Input: part model. Units: mm. Frame: model coordinates. Face numbers are marked on the shaded views. Coordinates: 2 decimals unless noted, no trailing zeros. Loops run counter-clockwise (first coordinate to the right, second up) from the corner with the lowest first, then second, coordinate; pieces in that order, holes last.
Item 1: Section B-B on x = 130.5. Return loops of the section in (y, z) (3 decimals).
Item 2: Section A-A on z = -22. Return loops of the section in (x, y) (3 decimals), and give its area (3 significant figures).
Item 3: Ray query, line 1 along X through (y, z) = (13.75, -50) (3 decimals); line 2 along X through (y, z) = (1.05, 0) (3 decimals); line 3 along Z through (x, y) = (141.5, 22.5) (3 decimals). Return the intervals inside material, ascending.
Item 4: Pull-direction query (X, two-part tool) for the marked faces 1 and 2; classes: released by +X, released by -X, zero draft, split by the parting line, or undercut.
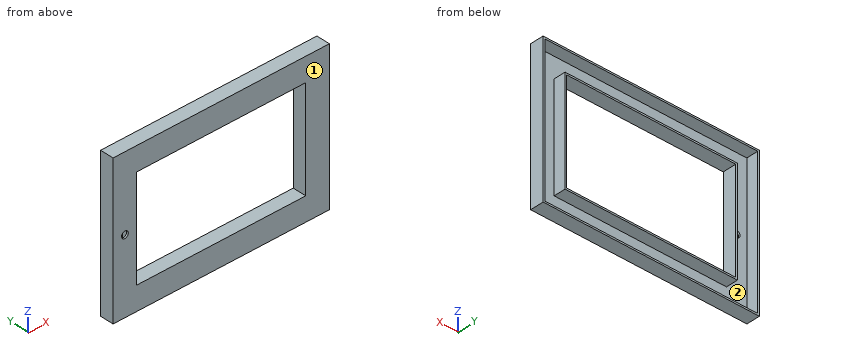
Autodesk Inventor part; units mm, degrees
ref_plane "YZ Plane" through (0, 0, 0) normal (1, 0, 0) x (0, 1, 0)
ref_plane "XZ Plane" through (0, 0, 0) normal (0, 1, 0) x (-1, 0, 0)
ref_plane "XY Plane" through (0, 0, 0) normal (0, 0, 1) x (1, 0, 0)
sketch "Sketch3" plane through (0, 0, 0) normal (0, 1, 0) x (-1, 0, 0)
  line L0 (-203.2, 139.7) -> (203.2, 139.7)
  line L1 (203.2, 139.7) -> (203.2, -139.7)
  line L2 (203.2, -139.7) -> (-203.2, -139.7)
  line L3 (-203.2, -139.7) -> (-203.2, 139.7)
  line L4 (-203.2, 139.7) -> (203.2, -139.7) construction
  line L5 (203.2, 139.7) -> (-203.2, -139.7) construction
  line L6 (152.4, -88.9) -> (152.4, 88.9)
  line L7 (152.4, 88.9) -> (-152.4, 88.9)
  line L8 (-152.4, 88.9) -> (-152.4, -88.9)
  line L9 (-152.4, -88.9) -> (152.4, -88.9)
  line L10 (158.75, -95.25) -> (158.75, 95.25)
  line L11 (158.75, 95.25) -> (-158.75, 95.25)
  line L12 (-158.75, 95.25) -> (-158.75, -95.25)
  line L13 (-158.75, -95.25) -> (158.75, -95.25)
  point P0 (0, 0)
  dimension "d11" = 406.4
  dimension "d12" = 279.4
  dimension "d13" = 50.8
  dimension "d14" = 44.45
extrude "Extrusion3" add sketch "Sketch3" along normal blind 50.8 contours L0 L1 L2 L3
shell "Shell2" thickness 3.175 removed faces 1 at (52.9167, 50.8, -124.8833)
sketch "Sketch4" plane through (0, 50.8, 0) normal (0, 1, 0) x (1, 0, 0)
  line L0 (227.9599, -165.6341) -> (-227.9599, -165.6341)
  line L1 (-227.9599, -165.6341) -> (-227.9599, 165.6341)
  line L2 (-227.9599, 165.6341) -> (227.9599, 165.6341)
  line L3 (227.9599, 165.6341) -> (227.9599, -165.6341)
  line L4 (227.9599, -165.6341) -> (-227.9599, 165.6341) construction
  line L5 (-227.9599, -165.6341) -> (227.9599, 165.6341) construction
  point P0 (0, 0)
extrude "Extrusion4" cut sketch "Sketch4" against normal blind 25.4
sketch "Sketch5" plane through (-200.025, 3.175, 136.525) normal (0, 1, 0) x (1, 0, 0)
  line L0 (361.95, 234.95) -> (38.1, 234.95)
  line L1 (361.95, 38.1) -> (361.95, 234.95)
  line L2 (38.1, 38.1) -> (361.95, 38.1)
  line L3 (38.1, 234.95) -> (38.1, 38.1)
  line L4 (400.05, 0) -> (0, 0)
  line L5 (400.05, 273.05) -> (400.05, 0)
  line L6 (0, 273.05) -> (400.05, 273.05)
  line L7 (0, 0) -> (0, 273.05)
  line L8 (38.1, 38.1) -> (0, 38.1)
  line L9 (0, 38.1) -> (0, 234.95)
  line L10 (0, 234.95) -> (38.1, 234.95)
  line L11 (38.1, 234.95) -> (38.1, 38.1)
  circle A0 centre (19.05, 136.525) radius 6.35
  point P0 (200.025, 136.525)
  dimension "d20" = 12.7
extrude "Extrusion5" cut sketch "Sketch5" against normal blind 25.4 contours A0
properties part number "Catch pan" material "Aluminum 6061"
Results found:
1. outline: (0, -139.7) - (25.4, -139.7) - (25.4, -136.525) - (3.175, -136.525) - (3.175, -98.425) - (25.4, -98.425) - (25.4, -95.25) - (0, -95.25) - close; (0, 95.25) - (25.4, 95.25) - (25.4, 98.425) - (3.175, 98.425) - (3.175, 136.525) - (25.4, 136.525) - (25.4, 139.7) - (0, 139.7) - close
2. outline: (-203.2, 0) - (-158.75, 0) - (-158.75, 25.4) - (-161.925, 25.4) - (-161.925, 3.175) - (-200.025, 3.175) - (-200.025, 25.4) - (-203.2, 25.4) - close; (158.75, 0) - (203.2, 0) - (203.2, 25.4) - (200.025, 25.4) - (200.025, 3.175) - (161.925, 3.175) - (161.925, 25.4) - (158.75, 25.4) - close
2. area: 565 mm2
3. line 1: x = -203.2 to -200.025, -161.925 to -158.75, 158.75 to 161.925, 200.025 to 203.2
3. line 2: x = -203.2 to -187.325, -174.625 to -158.75, 158.75 to 203.2
3. line 3: z = -139.7 to -136.525, -98.425 to -95.25, 95.25 to 98.425, 136.525 to 139.7
4. face 1: zero draft
4. face 2: undercut
